from build123d import *

# Parameters (mm, degrees)
BOSS_EXTRUDE1_DEPTH = 50


with BuildPart() as part:
    # Sketch1 → Boss-Extrude1 (new body)
    with BuildSketch(Plane.XY):
        with BuildLine():
            Line((-1, 41.98809355), (-1, 56.98809355))
            Line((-1, 56.98809355), (-3, 56.98809355))
            Line((-3, 56.98809355), (-3, 43.897608135))
            ThreePointArc((-3, 43.897608135), (-9.461252976, 42.97074228), (-15.714285714, 41.098190039))
            Line((-15.714285714, 41.098190039), (-15, 39.230090492))
            ThreePointArc((-15, 39.230090492), (-8.117982829, 41.207988968), (-1, 41.98809355))
        make_face()
    extrude(amount=BOSS_EXTRUDE1_DEPTH)


solid = part.part
Can you work these out from the model? Positions are in its coordinate system, mm. A direction names the side the tool comes from. Give positions to 0.01 mm unless a question says otherwise; leave off trailing zeros. Loops run counter-clockwise (first coordinate to the right, second up) from the corner with the lowest first, then second, coordinate; pieces in that order, holes last. Notation, with made-up numbers: M 0,3 L 52,3 A20 ccw 52,31 Z; hole C 9.25,15 d5. An arc over 180 degrees is marked long. One line per item, written item: value. Start each with the question number.
1) Thinking about a two-plate mould opening in X: for faces 3 (the face through (-4.6, 43.5, 50)), 4 (the face through (-8.216, 41.188, 24.65)), 5 (the face through (-15.362, 40.177, 24.65)), which applies, +X half, -X half, draft (parallel to the pull), parting line (faces both ways), or undercut?
2) If we section it at B-B, the plane y = 52: Write out the boundary of the cut face in (x, z), and give its area (3 significant figures).
3) If we section it at A-A, the plane z = 30: Write out the boundary of the cut face in (x, y), and give its area (3 significant figures).
4) If we section it at C-C, the plane x = -5.25: Write out the boundary of the cut face in (y, z).
5) I'm going to push flat-ended pins straight in: pin 1 (1.5 mm diameter, centred on x = -14, z = 29, fed in from -Y); pin 2 (2 mm diameter, centred on x = -13, z = 41.5, fed in from +Y); pin 3 (2 mm diameter, centred on x = -9, z = 11.5, fed in from +Y). Where does each tip first touch, or does it pass through?
6) On a 3-axis mill with a long thin cutter (end or side, diameter ignored), from which of +Z, -Z, +X, -X, +Y, -Y can I reach the whole of each face in a straight line? I mean faces 1 (the face through (-1, 49, 25)), 2 (the face through (-3, 51, 25)). Say none if no direction works.
7) If I drill on line 1 (X direction, y = 50.75, z = 12); line 2 (Y direction, x = -1.25, z = 17); line 3 (Y direction, x = -7.25, z = 12.5), over which ranges is the centre line in solid material (lowest first)? Write a range as [from, to].
Completed:
1. face 3: draft
1. face 4: +X half
1. face 5: -X half
2. outline: M -3,0 L -1,0 L -1,50 L -3,50 Z
2. area: 100 mm^2
3. outline: M -15.71,41.1 L -15,39.23 A42 cw -1,41.99 L -1,56.99 L -3,56.99 L -3,43.9 A44 ccw Z
3. area: 55.5 mm^2
4. outline: M 41.67,0 L 43.69,0 L 43.69,50 L 41.67,50 Z
5. pin 1: stops at y = 39.32
5. pin 2: stops at y = 42.33
5. pin 3: stops at y = 43.27
6. face 1: +Z, -Z, +X, +Y, -Y
6. face 2: +Z, -Z, -X, +Y
7. line 1: x = [-3, -1]
7. line 2: y = [41.98, 56.99]
7. line 3: y = [41.37, 43.4]
